Autodesk Inventor part; units mm, degrees
ref_plane "Work Plane2" through (-30, -30, -120) normal (0, 1, 0) x (1, 0, 0)
ref_plane "Work Plane6" through (-7.5, -30, -10) normal (0, 0, -1) x (-1, 0, 0)
ref_plane "YZ Plane" through (0, 0, 0) normal (1, 0, 0) x (0, 1, 0)
sketch "Sketch1" plane through (0, 0, 0) normal (0, 1, 0) x (-1, 0, 0)
  line L0 (0, 0) -> (60, 0)
  line L1 (60, 0) -> (60, -120)
  line L2 (60, -120) -> (0, -120)
  line L3 (0, -120) -> (0, 0)
  line L4 (30, -120) -> (30, 0)
  circle A0 centre (30, -55) radius 22.5
  line L5 (19.5, -90) -> (19.5, -115)
  line L6 (19.5, -115) -> (40.5, -115)
  line L7 (40.5, -115) -> (40.5, -90)
  line L8 (40.5, -90) -> (19.5, -90)
  line L9 (19.5, -90) -> (40.5, -115) construction
  line L10 (19.5, -115) -> (40.5, -90) construction
  line L11 (19.5, -90) -> (44.5, -90) construction
  line L12 (25, -80) -> (25, -90)
  line L13 (25, -90) -> (35, -90)
  line L14 (35, -90) -> (35, -80)
  line L15 (35, -80) -> (25, -80)
  line L16 (25, -80) -> (35, -90) construction
  line L17 (25, -90) -> (35, -80) construction
  line L18 (25, -80) -> (35, -80) construction
  line L19 (7.5, -10) -> (7.5, -80)
  line L20 (7.5, -80) -> (52.5, -80)
  line L21 (52.5, -80) -> (52.5, -10)
  line L22 (52.5, -10) -> (7.5, -10)
  line L23 (7.5, -10) -> (52.5, -80) construction
  line L24 (7.5, -80) -> (52.5, -10) construction
  line L25 (7.5, -10) -> (77.5, -10) construction
  point P0 (30, -115)
  point P1 (30, -90)
  point P2 (30, -90)
  point P3 (30, -80)
  point P4 (30, -77.5)
  point P5 (30, -25)
  point P6 (30, -102.5)
  point P7 (30, -10)
  point P8 (30, -85)
  point P9 (30, -10)
  point P10 (30, -45)
  point P11 (25, -90)
  point P12 (35, -90)
  point P13 (35, -80)
  point P14 (25, -80)
  dimension "d0" = 60
  dimension "d1" = 120
  dimension "d2" = 45
  dimension "d3" = 5
  dimension "d4" = 25
  dimension "d5" = 0
  dimension "d6" = 12.5
  dimension "d7" = 10
  dimension "d8" = 2.5
  dimension "d9" = 22.5
  dimension "d10" = -70
  dimension "d11" = 25
  dimension "d12" = 90
  dimension "d13" = 21
  dimension "d14" = 5
  dimension "d15" = 10
  dimension "d16" = 90
  dimension "d17" = 10
  dimension "d19" = -70
  dimension "d20" = 90
  dimension "d21" = -35
  dimension "d22" = 45
extrude "Extrusion1" add sketch "Sketch1" along normal blind 20
ref_plane "Work Plane1" through (0, 20, -120) normal (0, 0, -1) x (-1, 0, 0)
sketch "Sketch2" plane through (0, 20, -120) normal (0, 0, -1) x (-1, 0, 0)
  line L0 (0, -20) -> (60, -20)
  line L1 (60, -20) -> (60, 0)
  line L2 (0, 0) -> (60, 0)
  line L3 (0, -20) -> (0, 0)
  line L4 (60, -20) -> (0, -20)
  line L5 (0, -20) -> (60, -20)
  line L6 (60, -20) -> (60, -80)
  line L7 (60, -80) -> (0, -80)
  line L8 (0, -80) -> (0, -20)
  point P0 (30, -50)
  dimension "d25" = 60
  dimension "d26" = 60
  dimension "d27" = 30
  dimension "d28" = 30
ref_plane "Work Plane2" through (-30, -30, -120) normal (0, 1, 0) x (1, 0, 0)
extrude "Extrusion2" add sketch "Sketch1" against normal up to surface (30 mm away) contours L22 L21 A0 L4 | L4 A0 L19 L22 | A0 L4 | L4 A0 | L6 L5 L8 L4 | L4 L8 L7 L6 | A0 L21 L20 L15 L4 | L4 L15 L20 L19 A0 | L8 L12 L15 L4 | L4 L15 L14 L8
extrude "Extrusion3" cut sketch "Sketch1" along normal through all both and the other way through all contours A0 L4 | L4 A0
ref_plane "Work Plane6" through (-7.5, -30, -10) normal (0, 0, -1) x (-1, 0, 0)
ref_plane "Work Plane5" through (-7.5, -30, -80) normal (0, 0, -1) x (-1, 0, 0)
sketch "Sketch3" plane through (-40.5, -30, -115) normal (0, 0, -1) x (-1, 0, 0)
  line L0 (0, 30) -> (0, 0)
  circle A0 centre (-10.5, 0) radius 10.5
  point P0 (-40.5, 30)
sketch "Sketch4" plane through (-19.5, -30, -90) normal (0, 0, -1) x (-1, 0, 0)
  line L0 (5.5, 30) -> (5.5, 0)
  line L1 (15.5, 30) -> (15.5, 0)
  circle A0 centre (10.5, 0) radius 5
  point P0 (-19.5, 30)
sketch "Sketch5" plane through (-7.5, -30, -80) normal (0, 0, -1) x (-1, 0, 0)
  line L0 (0, 50) -> (45, 50)
  circle A0 centre (22.5, 0) radius 22.5
  point P0 (-7.5, 30)
extrude "Extrusion4" cut sketch "Sketch3" against normal up to surface (25 mm away)
extrude "Extrusion5" cut sketch "Sketch5" against normal up to surface (70 mm away)
extrude "Extrusion6" cut sketch "Sketch4" against normal up to surface (10 mm away)
ref_plane "Work Plane3" through (-40.5, -30, -115) normal (0, 0, -1) x (-1, 0, 0)
ref_plane "Work Plane4" through (-19.5, -30, -90) normal (0, 0, -1) x (-1, 0, 0)
equation "\"d19\" = d10"
equation "\"d22\" = d2"
equation "\"d25\" = d0"
equation "\"d26\" = d25"
properties part number "housing_lid_V2"
Can you work these out from the model? Positions are in its coordinate system, mm. A direction names the side the tool comes from. Give positions to 0.01 mm unless a question says otherwise; leave off trailing zeros. Write each loop counter-clockwise with the first axis right and the second up, starting at its lowest first coordinate (ties: lowest second). Pieces come first, ordered by that corner, then holes. Notation, with made-up numbers: (54, 21.5) -> (109, 21.5) arc R29 cw to (109, 41.5) -> close; hole circle Ø4 at (-23, -35). An arc over 180 degrees is marked (long way). One line per item, written item: value.
Q1. For P1, Ø15, axis at y = -19, z = -22, coming from the -X side; P2, Ø5, axis at x = -29.5, y = -26, coming from the -Z side; P3, Ø12.5, axis at y = -19.5, z = -96.5, coming from the -X side; P4, Ø6, axis at x = -15.5, y = -18.5, coming from the +Z side, each with a flat end and sliding along its axis, tell me the tip position at first contact or that it passes through.
Results found:
P1: stops at x = -52.5
P2: stops at z = -90
P3: stops at x = -40.5
P4: passes through
Q2. Imagine slicing it at B-B on x = -30. Please give me the cut outline in (y, z), and give its area (4 significant figures).
Results found:
outline: (-25, -90) -> (-19.5, -90) -> (-19.5, -115) -> (0, -115) -> (0, -120) -> (20, -120) -> (20, -77.5) -> (-7.5, -77.5) -> (-7.5, -80) -> (-25, -80) -> close; (-7.5, -32.5) -> (20, -32.5) -> (20, 0) -> (0, 0) -> (0, -10) -> (-7.5, -10) -> close
area: 2,425 mm^2
Q3. Imagine slicing it at C-C on z = -56.5. Please give me the cut outline in (x, y).
Results found:
outline: (-60, 0) -> (-52.5, 0) -> (-52.5, -30) arc R22.5 cw to (-52.45, -28.5) -> (-52.45, 20) -> (-60, 20) -> close; (-7.55, -28.5) arc R22.5 cw to (-7.5, -30) -> (-7.5, 0) -> (0, 0) -> (0, 20) -> (-7.55, 20) -> close
Q4. Which directions (+Z, -Z, +X, -X, +Y, -Y) give clear straight access to the entire face, cutting with the end or side of a thin tool? Please do faces 1 (the face through (-30, -5, -10)), 2 (the face through (-46, -8, -80)), 3 (the face through (-7.5, -15, -45)).
Results found:
face 1: +Z, +X, -X, -Y
face 2: -X, -Y
face 3: +Z, -Z, +X, -Y
Q5. We'd pull the mould along X, two halves only. Please class faces 4 (the face through (-30, 10, 0)), 5 (the face through (-30.495, -7.505, -27.815)), 6 (the face through (-40.5, -15, -103)), 7 (the face through (-19.5, -15, -102)): +X half, -X half, draft (parallel to the pull), parting line (faces both ways), or undercut.
Results found:
face 4: draft
face 5: undercut
face 6: -X half
face 7: +X half
Q6. Imagine slicing it at D-D on y = 8.5. Please give me the cut outline in (x, z), and give its area (3 significant figures).
Results found:
outline: (-60, -120) -> (0, -120) -> (0, 0) -> (-60, 0) -> close; hole circle Ø45 at (-30, -55)
area: 5,610 mm^2
Q7. Please list where these lines run through material, in increasing order: line 1 (X direction, y = 1, z = -55); line 2 (Y direction, x = -58, z = -23); line 3 (Z direction, x = -38, y = -2). Write a range as [from, to].
Results found:
line 1: x = [-60, -52.5], [-7.5, 0]
line 2: y = [0, 20]
line 3: z = [-115, -90], [-80, -76.03], [-33.97, -10]
